```python
from build123d import *

# Parameters (mm, degrees)
ESQUISSE1_R        = 18
ESQUISSE1_R_2      = 3
BOSS_EXTRU_1_DEPTH = 3
ESQUISSE2_R        = 13
ESQUISSE2_R_2      = 3
BOSS_EXTRU_2_DEPTH = 3
CHANFREIN1_SIZE    = 5


with BuildPart() as part:
    # Esquisse1 → Boss.-Extru.1 (new body)
    with BuildSketch(Plane.XY):
        Circle(ESQUISSE1_R)
        Circle(ESQUISSE1_R_2, mode=Mode.SUBTRACT)
    extrude(amount=BOSS_EXTRU_1_DEPTH)

    # Esquisse2 → Boss.-Extru.2 (add)
    with BuildSketch(Plane.XY.offset(3)):
        Circle(ESQUISSE2_R)
        Circle(ESQUISSE2_R_2, mode=Mode.SUBTRACT)
    extrude(amount=BOSS_EXTRU_2_DEPTH)

    # Chanfrein1
    # the kernel refuses this chamfer: 5 mm, written as the material it takes off along each edge
    with BuildSketch(Plane(origin=(0, 0, 6), x_dir=(1, 0, 0), z_dir=(0, -1, 0))) as chanfrein1_piece_1_section:
        Polygon((13, -CHANFREIN1_SIZE), (13 - CHANFREIN1_SIZE, 0), (13, 0), align=None)
    chanfrein1_piece_1 = revolve(axis=Axis((0, 0, 6), (0, 0, 1)), mode=Mode.PRIVATE)
    chanfrein1_piece_1 = split(chanfrein1_piece_1, bisect_by=Plane(origin=(-9.494850826, 0, 3), z_dir=(0, 0, 1)), keep=Keep.TOP, mode=Mode.PRIVATE)
    add(chanfrein1_piece_1, mode=Mode.SUBTRACT)


solid = part.part
```
Here's how the part is built. I have some questions about the finished solid (model axes, mm). Coordinates: 2 decimals unless noted, no trailing zeros. Write each loop counter-clockwise with the first axis right and the second up, starting at its lowest first coordinate (ties: lowest second). Pieces come first, ordered by that corner, then holes. Notation, with made-up numbers: M 82.25,28.25 L 110.25,28.25 A15 ccw 110.25,51.25 Z; hole C 45.5,63.25 d2. An arc over 180 degrees is marked long. Answer as CSV lines item,"result". Start each with the question number.
Q1. Suppose I cut it at A-A, the plane x = 0. List the corners of the cut face in (y, z) for me.
Q2. If we mould it in two halves opening along X, with no side actions, what happens to faces 1 (the cylindrical face through (-3, 0, 3)), 2 (the conical face through (-1.766, -7.952, 5.854)), 3 (the flat face through (-8, -8, 3))? For each: pulls with the +X half, pulls with the -X half, needs draft (parallel to the pull), parting line crosses it, or undercut.
Q3. Suppose I cut it at B-B, the plane z = 1.5. List the corners of the cut face in (x, y) for me, then the cut area to 3 significant figures.
Q4. Will these pins go through, and if not, where does the flat tip stop? pin 1 Ø2 at (x, z) = (-2, 1.5) entering from +Y; pin 2 Ø2 at (x, z) = (2, 1) entering from -Y; pin 3 Ø1.5 at (x, z) = (10, 5.5) entering from +Y.
Q5. Suppose I cut it at C-C, the plane y = 12. List the corners of the cut face in (x, z) for me, then the cut area to 3 significant figures.
Q6. I need wall thicknesses on probe 1 along Y at (x, z) = (0, 4.1); probe 2 along X at (y, z) = (1, 4.25); probe 3 along Y at (x, z) = (0, 3.85). Which ranges of each line are inside material? Lowest first, please. Write a range as [from, to].
Q7. Suppose I cut it at D-D, the plane z = 4.5. List the corners of the cut face in (x, y) for me, then the cut area to 3 significant figures.
Entries:
1,outline,"M -18,0 L -3,0 L -3,6 L -8,6 L -11,3 L -18,3 Z; M 3,0 L 18,0 L 18,3 L 11,3 L 8,6 L 3,6 Z"
2,face 1,"undercut"
2,face 2,"parting line crosses it"
2,face 3,"needs draft"
3,outline,"C 0,0 d36; hole C 0,0 d6"
3,area,"990 mm²"
4,pin 1,"stops at y = 17.97"
4,pin 2,"stops at y = -17.97"
4,pin 3,"passes through"
5,outline,"M -13.42,0 L 13.42,0 L 13.42,3 L -13.42,3 Z"
5,area,"80.5 mm²"
6,probe 1,"y = [-9.9, -3], [3, 9.9]"
6,probe 2,"x = [-9.7, -2.83], [2.83, 9.7]"
6,probe 3,"y = [-10.15, -3], [3, 10.15]"
7,outline,"C 0,0 d19; hole C 0,0 d6"
7,area,"255 mm²"
